Check sheet for the modelled part. Datum: model origin and axes. Units: mm. Face numbers are marked on the shaded views. A direction names the side the tool comes from. Give positions to 0.01 mm unless a question says otherwise; leave off trailing zeros. Loops run counter-clockwise (first coordinate to the right, second up) from the corner with the lowest first, then second, coordinate; pieces in that order, holes last. Notation, with made-up numbers: M 71,83.25 L 103,83.25 A19 cw 103,99.25 Z; hole C -35.5,62.25 d8. An arc over 180 degrees is marked long. One line per question, with ' | ' between items. Start each with the question number.
from build123d import *

# Parameters (mm, degrees)
SKETCH_1_R               = 6
EXTRUDE_1_DEPTH          = 15
FILLET_1_R               = 8
FILLET_2_R               = 8
FILLET_3_R               = 5
EXTRUDE_3_DEPTH          = 60
CUT_EXTRUDE_START        = -20
SKETCH_5_R               = 18
CUT_EXTRUDE_1_DEPTH      = 20
CUT_EXTRUDE_START_2      = -15
CUT_EXTRUDE_2_DEPTH      = 15
CUT_EXTRUDE_3_REACH      = 168.283
CUT_EXTRUDE_3_END_RADIUS = 18
SKETCH_7_R               = 6
EXTRUDE_4_DEPTH          = 10


with BuildPart() as part:
    # 草图1 → 凸台-拉伸1 (new body)
    with BuildSketch(Plane(origin=(0, 0, 0), x_dir=(1, 0, 0), z_dir=(0, 1, 0))):
        Polygon((0, 0), (0, -65), (22.5, -65), (22.5, -80), (102.5, -80), (102.5, -63.32326284), (125, -63.32326284), (125, 0), align=None)
        with Locations(Location((14.5, -51, 0), (0, 0, 270))):
            Circle(SKETCH_1_R, mode=Mode.SUBTRACT)
        with Locations(Location((110.5, -51, 0), (0, 0, 270))):
            Circle(SKETCH_1_R, mode=Mode.SUBTRACT)
    extrude(amount=EXTRUDE_1_DEPTH)

    # 圆角1
    fillet_1_edges = [part.edges().sort_by_distance(p)[0] for p in [
        (125, 7.5, 63.32326284),
        (0, 7.5, 65),
    ]]
    fillet(fillet_1_edges, radius=FILLET_1_R)

    # 圆角2
    fillet_2_edges = [part.edges().sort_by_distance(p)[0] for p in [
        (102.5, 7.5, 80),
        (22.5, 7.5, 80),
    ]]
    fillet(fillet_2_edges, radius=FILLET_2_R)

    # 圆角3
    fillet_3_edges = [part.edges().sort_by_distance(p)[0] for p in [
        (102.5, 7.5, 63.32326284),
        (22.5, 7.5, 65),
    ]]
    fillet(fillet_3_edges, radius=FILLET_3_R)

    # 草图2 → 凸台-拉伸3 (add)
    with BuildSketch(Plane(origin=(0, 15, 0), x_dir=(1, 0, 0), z_dir=(0, 1, 0))):
        with BuildLine():
            Line((95.5, 0), (62.5, 0))
            Line((62.5, 0), (62.5, -17))
            ThreePointArc((62.5, -17), (75.227922061, -22.272077939), (80.5, -35))
            Line((80.5, -35), (95.5, -35))
            Line((95.5, -35), (95.5, 0))
        make_face()
        with BuildLine():
            Line((62.5, -17), (62.5, 0))
            Line((62.5, 0), (29.5, 0))
            Line((29.5, 0), (29.5, -35))
            Line((29.5, -35), (44.5, -35))
            ThreePointArc((44.5, -35), (49.772077939, -22.272077939), (62.5, -17))
        make_face()
        with BuildLine():
            Line((95.5, -35), (80.5, -35))
            ThreePointArc((80.5, -35), (62.5, -53), (44.5, -35))
            Line((44.5, -35), (29.5, -35))
            ThreePointArc((29.5, -35), (62.5, -68), (95.5, -35))
        make_face()
    extrude(amount=EXTRUDE_3_DEPTH)

    # 草图5 → 切除-拉伸1 (cut)
    with BuildSketch(Plane(origin=(0, 75, 0), x_dir=(1, 0, 0), z_dir=(0, 1, 0)).offset(CUT_EXTRUDE_START)):
        with Locations((62.5, -35)):
            Circle(SKETCH_5_R)
        with BuildLine():
            Line((29.5, -35), (95.5, -35))
            ThreePointArc((95.5, -35), (62.5, -68), (29.5, -35))
        make_face()
    extrude(amount=CUT_EXTRUDE_1_DEPTH, mode=Mode.SUBTRACT)

    # 草图6 → 切除-拉伸2 (cut)
    with BuildSketch(Plane(origin=(0, 55, 0), x_dir=(1, 0, 0), z_dir=(0, 1, 0)).offset(CUT_EXTRUDE_START_2)):
        with BuildLine():
            Line((56.5, -51.970562748), (56.5, -67.449961479))
            ThreePointArc((56.5, -67.449961479), (59.487420442, -67.862202671), (62.5, -68))
            Line((62.5, -68), (62.5, -53))
            ThreePointArc((62.5, -53), (59.456164383, -52.740774074), (56.5, -51.970562748))
        make_face()
        with BuildLine():
            Line((62.5, -53), (62.5, -68))
            ThreePointArc((62.5, -68), (65.512579558, -67.862202671), (68.5, -67.449961479))
            Line((68.5, -67.449961479), (68.5, -51.970562748))
            ThreePointArc((68.5, -51.970562748), (65.543835617, -52.740774074), (62.5, -53))
        make_face()
    extrude(amount=CUT_EXTRUDE_2_DEPTH, mode=Mode.SUBTRACT)

    # 切除-拉伸3: up to this cylinder (the profile starts outside it)
    cut_extrude_3_end = Plane(origin=(62.5, 55, 35), z_dir=(0, -1, 0)) * Cylinder(CUT_EXTRUDE_3_END_RADIUS, 373.566, mode=Mode.PRIVATE)
    # 草图7 → 切除-拉伸3 (cut, up to the surface)
    with BuildSketch(Plane(origin=(0, 0, 0), x_dir=(-1, 0, 0), z_dir=(0, 0, -1)), mode=Mode.PRIVATE) as cut_extrude_3_sk1:
        with Locations((-62.5, 55)):
            Circle(SKETCH_7_R)
    cut_extrude_3_tool1 = extrude(cut_extrude_3_sk1.sketch, amount=-CUT_EXTRUDE_3_REACH, mode=Mode.PRIVATE) - cut_extrude_3_end
    add(cut_extrude_3_tool1.solids().sort_by_distance((62.5, 55, 0))[0], mode=Mode.SUBTRACT)

    # 草图10 → 凸台-拉伸4 (add)
    with BuildSketch(Plane(origin=(0, 0, 30), x_dir=(-1, 0, 0), z_dir=(0, 0, -1))):
        Polygon((-95.5, 15), (-105.5, 15), (-95.5, 35), align=None)
        Polygon((-19.5, 15), (-29.5, 35), (-29.5, 15), align=None)
    extrude(amount=-EXTRUDE_4_DEPTH)


solid = part.part
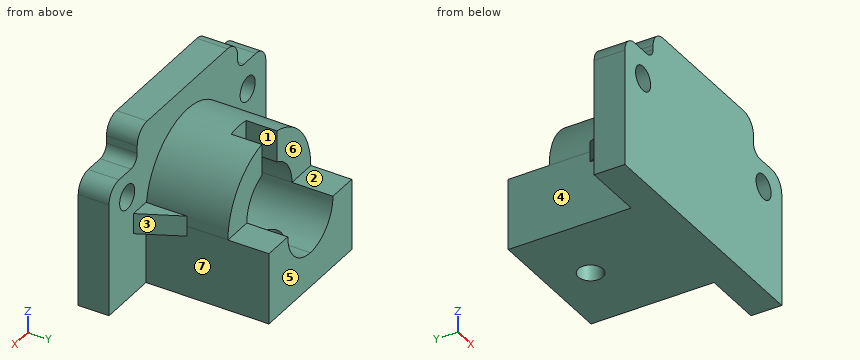
Q1. Draft check along X on the marked faces 1, 2, 3 and 4. Enter one of: released by +X, released by -X, zero draft, split by the parting line, or undercut.
Q2. Cross-section at B-B (y = 62.5). Record the cut outline in (x, z), and give its area (3 significant figures).
Q3. Material ranges on probe 1 along X at (y, z) = (9.25, 51); probe 2 along Z at (x, y) = (110, 3); probe 3 along Y at (x, z) = (62, 14), recorded low to high. Write a range as from..to.
Q4. Cross-section at A-A (x = 110.5). Record the cut outline in (y, z).
Q5. Cross-section at C-C (z = 12). Record the cut outline in (x, y), and give its area (3 significant figures).
Q6. Cross-section at D-D (y = 23.5). Record the cut outline in (x, z), and give its area (3 significant figures).
Q7. Depth check by flat-ended pin: P1, Ø3, axis at x = 77, z = 62.5, coming from the +Y side; P2, Ø0.6, axis at y = 9, z = 70.5, coming from the -X side; P3, Ø5, axis at x = 110.5, y = 7, coming from the +Z side. Enter the tip coordinate at first touch or a pass-through.
Q8. Access from +Z, -Z, +X, -X, +Y, -Y to the whole of each face (thin tool, end or side, straight path). Record for the marked faces 5, 6 and 7.
Solved:
1) face 1: undercut | face 2: zero draft | face 3: released by +X | face 4: released by -X
2) outline: M 29.5,0 L 95.5,0 L 95.5,35 L 80.5,35 A18 cw 44.5,35 L 29.5,35 Z | area: 1,800 mm²
3) probe 1: x = 0..8.5, 20.5..104.5, 116.5..125 | probe 2: z = 0..45.02, 56.98..63.32 | probe 3: y = 0..49.02, 60.98..75
4) outline: M 0,0 L 15,0 L 15,45 L 0,45 Z; M 0,57 L 15,57 L 15,63.32 L 0,63.32 Z
5) outline: M 0,0 L 125,0 L 125,15 L 95.5,15 L 95.5,75 L 29.5,75 L 29.5,15 L 0,15 Z; hole C 62.5,55 d12 | area: 5,720 mm²
6) outline: M 23.75,30 L 29.5,30 L 29.5,0 L 95.5,0 L 95.5,30 L 101.25,30 L 101.25,40 L 95.5,40 L 95.5,35 A33 ccw 29.5,35 L 29.5,40 L 23.75,40 Z; hole C 62.5,35 d36 | area: 3,120 mm²
7) P1: stops at y = 55 | P2: stops at x = 22.5 | P3: stops at z = 63.32
8) face 5: +Z, -Z, +X, -X, +Y | face 6: +Z, +X, -X, +Y | face 7: -Z, +X, +Y
